Geometry: final body of the model. Coordinates: model frame, mm. Give positions to 0.01 mm unless a question says otherwise; leave off trailing zeros. Loops run counter-clockwise (first coordinate to the right, second up) from the corner with the lowest first, then second, coordinate; pieces in that order, holes last. Notation, with made-up numbers: (37.25, 59.5) -> (47.25, 59.5) arc R9 cw to (47.25, 69.5) -> close; hole circle Ø7 at (36, 2). An arc over 180 degrees is marked (long way). Answer in a Markdown table with one row per item. Add a question column.
1) Section query A-A (y = 2.9). Return the cut outline in (x, z).
2) Line query: line 1 (X direction, y = 4.7, z = 20); line 2 (Y direction, x = 7, z = 25). Output: solid intervals per line, ascending. Write a range as from..to.
3) First-contact query: P1, Ø2, axis at x = 5, y = 2, coming from the -Z side. Flat tip, straight axial feed; report the tip coordinate or a pass-through.
4) Section query C-C (z = 0.5). Return the cut outline in (x, y).
5) Section query B-B (x = 2.25). Return the cut outline in (y, z), plus the area to 3 significant figures.
Autodesk Inventor part; units mm, degrees
ref_plane "YZ Plane" through (0, 0, 0) normal (1, 0, 0) x (0, 1, 0)
ref_plane "XZ Plane" through (0, 0, 0) normal (0, 1, 0) x (-1, 0, 0)
ref_plane "XY Plane" through (0, 0, 0) normal (0, 0, 1) x (1, 0, 0)
sketch "Sketch1" plane through (0, 0, 0) normal (0, 1, 0) x (-1, 0, 0)
  line L0 (-10.3, 50) -> (10.3, 50)
  line L1 (10.3, 50) -> (10.3, -50)
  line L2 (10.3, -50) -> (-10.3, -50)
  line L3 (-10.3, -50) -> (-10.3, 50)
  line L4 (-10.3, 50) -> (10.3, -50) construction
  line L5 (10.3, 50) -> (-10.3, -50) construction
  point P0 (0, 0)
  dimension "d0" = 100
  dimension "d1" = 20.6
extrude "Extrusion1" add sketch "Sketch1" along normal blind 5.6
sketch "Sketch2" plane through (-10.3, 0, 50) normal (0, 0, 1) x (1, 0, 0)
  line L0 (0.3, 0.3) -> (20.3, 0.3)
  line L1 (20.3, 0.3) -> (20.3, 5.3)
  line L2 (20.3, 5.3) -> (0.3, 5.3)
  line L3 (0.3, 5.3) -> (0.3, 0.3)
  line L4 (0, 0) -> (20.6, 0)
  line L5 (0, 5.6) -> (20.6, 5.6)
  line L6 (20.6, 0) -> (20.6, 5.6)
  line L7 (0, 0) -> (0, 5.6)
  point P0 (10.3, 0)
  dimension "d4" = 0.3
  dimension "d5" = 0.3
  dimension "d6" = 0.3
  dimension "d7" = 0.3
extrude "Extrusion2" cut sketch "Sketch2" against normal through all contours L3 L2 L1 L0
fillet "Fillet1" radius 0.05 4 edges at (-10.3, 5.6, 0) (-10.3, 0, 0) (10, 5.3, 0) (10.3, 0, 0)
properties part number "RubberPiece"
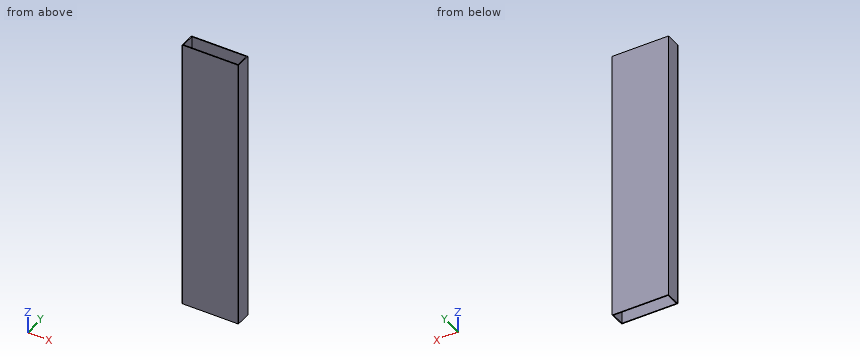
Evaluation:
| question | item | result |
|---|---|---|
| 1 | outline | (-10.3, -50) -> (-10, -50) -> (-10, 50) -> (-10.3, 50) -> close; (10, -50) -> (10.3, -50) -> (10.3, 50) -> (10, 50) -> close |
| 2 | line 1 | -10.3..-10, 10..10.3 |
| 2 | line 2 | 0..0.3, 5.3..5.6 |
| 3 | P1 | through |
| 4 | outline | (-10.3, 0.05) arc R0.05 ccw to (-10.25, 0) -> (10.25, 0) arc R0.05 ccw to (10.3, 0.05) -> (10.3, 5.6) -> (-10.25, 5.6) arc R0.05 ccw to (-10.3, 5.55) -> close; hole (-10, 0.3) -> (10, 0.3) -> (10, 5.25) arc R0.05 ccw to (9.95, 5.3) -> (-10, 5.3) -> close |
| 5 | outline | (0, -50) -> (0.3, -50) -> (0.3, 50) -> (0, 50) -> close; (5.3, -50) -> (5.6, -50) -> (5.6, 50) -> (5.3, 50) -> close |
| 5 | area | 60.0 mm² |
